Input: part model. Units: mm. Frame: model coordinates. A direction names the side the tool comes from. Round coordinates to 2 decimals unless told otherwise and drop trailing zeros. Write each loop counter-clockwise with the first axis right and the second up, starting at its lowest first coordinate (ties: lowest second). Pieces come first, ordered by that corner, then holes. Notation, with made-up numbers: (76.25, -13) -> (120.25, -13) arc R9 cw to (120.25, -4) -> close; hole circle Ø10 at (-35.5, 53.5). An arc over 180 degrees is marked (long way). Write item = value, one per line.
```python
from build123d import *

# Parameters (mm, degrees)
SKETCH1_R           = 5
BOSS_EXTRUDE1_DEPTH = 20
SKETCH2_R           = 2.5
CUT_EXTRUDE1_DEPTH  = 21
BOSS_EXTRUDE2_DEPTH = 18
SKETCH5_R           = 7.5
SKETCH5_R_2         = 2.5
BOSS_EXTRUDE3_DEPTH = 1
SKETCH4_R           = 7.5
BOSS_EXTRUDE4_DEPTH = 1
SKETCH7_R           = 0.5
CUT_EXTRUDE2_DEPTH  = 2


with BuildPart() as part:
    # Sketch1 → Boss-Extrude1 (new body)
    with BuildSketch(Plane(origin=(0, 0, 0), x_dir=(1, 0, 0), z_dir=(0, 1, 0))):
        with Locations(Location((0, 0, 0), (0, 0, 270))):  # turned: the seam where the file's is
            Circle(SKETCH1_R)
    extrude(amount=BOSS_EXTRUDE1_DEPTH)

    # Sketch2 → Cut-Extrude1 (cut, through all)
    with BuildSketch(Plane(origin=(0, 20, 0), x_dir=(1, 0, 0), z_dir=(0, 1, 0))):
        with Locations(Location((0, 0, 0), (0, 0, 270))):  # turned: the seam where the file's is
            Circle(SKETCH2_R)
    extrude(amount=-CUT_EXTRUDE1_DEPTH, mode=Mode.SUBTRACT)

    # Sketch3 → Boss-Extrude2 (add)
    with BuildSketch(Plane(origin=(0, 20, 0), x_dir=(1, 0, 0), z_dir=(0, 1, 0))):
        with BuildLine():
            Line((1.5, -2), (-1.5, -2))
            ThreePointArc((-1.5, -2), (0, -2.5), (1.5, -2))
        make_face()
    extrude(amount=-BOSS_EXTRUDE2_DEPTH)

    # Sketch5 → Boss-Extrude3 (add)
    with BuildSketch(Plane.XZ):
        with Locations(Location((0, 0, 0), (0, 0, 270))):  # turned: the seam where the file's is
            Circle(SKETCH5_R)
        with Locations(Location((0, 0, 0), (0, 0, 90))):  # turned: the seam where the file's is
            Circle(SKETCH5_R_2, mode=Mode.SUBTRACT)
    extrude(amount=-BOSS_EXTRUDE3_DEPTH)

    # Sketch4 → Boss-Extrude4 (add)
    with BuildSketch(Plane(origin=(0, 20, 0), x_dir=(1, 0, 0), z_dir=(0, 1, 0))):
        with Locations(Location((0, 0, 0), (0, 0, 90))):  # turned: the seam where the file's is
            Circle(SKETCH4_R)
        with BuildLine():
            Line((1.5, -2), (-1.5, -2))
            ThreePointArc((-1.5, -2), (0, 2.5), (1.5, -2))
        make_face(mode=Mode.SUBTRACT)
    extrude(amount=-BOSS_EXTRUDE4_DEPTH)

    # Sketch7 → Cut-Extrude2 (cut, through all)
    with BuildSketch(Plane.XZ.offset(-19)):
        with Locations(Location((-2.100852557, 5.628196829, 0), (0, 0, 270))):  # turned: the seam where the file's is
            Circle(SKETCH7_R)
    extrude(amount=-CUT_EXTRUDE2_DEPTH, mode=Mode.SUBTRACT)


solid = part.part
```
1) Cut plane B-B (z = 0). Return the cut outline in (x, y).
Solutions:
outline = (-7.5, 0) -> (-2.5, 0) -> (-2.5, 20) -> (-7.5, 20) -> (-7.5, 19) -> (-5, 19) -> (-5, 1) -> (-7.5, 1) -> close; (2.5, 0) -> (7.5, 0) -> (7.5, 1) -> (5, 1) -> (5, 19) -> (7.5, 19) -> (7.5, 20) -> (2.5, 20) -> close
2) Cut plane A-A (x = 0). Return the cut outline in (y, z).
Solutions:
outline = (0, -7.5) -> (1, -7.5) -> (1, -5) -> (19, -5) -> (19, -7.5) -> (20, -7.5) -> (20, -2.5) -> (0, -2.5) -> close; (0, 2.5) -> (2, 2.5) -> (2, 2) -> (20, 2) -> (20, 7.5) -> (19, 7.5) -> (19, 5) -> (1, 5) -> (1, 7.5) -> (0, 7.5) -> close
3) Cut plane C-C (y = 15). Return the cut outline in (x, z), and give its area (3 significant figures).
Solutions:
outline = circle Ø10 at (0, 0); hole (-1.5, 2) arc R2.5 ccw (long way) to (1.5, 2) -> close
area = 59.9 mm^2
4) Access query for faces 5 (the face through (-4.88, 9.87, -1.08)), 6 (the face through (0, 11, 2)), 7 (the face through (2, 0, 2)). Directions: +Z, -Z, +X, -X, +Y, -Y. A direction counts if a zero-diameter tool reaches every point of the face in a straight line with its end or side. Return the directions, or none.
Solutions:
face_5 = none
face_6 = +Y, -Y
face_7 = +Z, -Z, +X, -X, -Y
5) Cut plane D-D (x = 4.25). Return the cut outline in (y, z), and give its area (3 significant figures).
Solutions:
outline = (0, -6.18) -> (1, -6.18) -> (1, -2.63) -> (19, -2.63) -> (19, -6.18) -> (20, -6.18) -> (20, 6.18) -> (19, 6.18) -> (19, 2.63) -> (1, 2.63) -> (1, 6.18) -> (0, 6.18) -> close
area = 120 mm^2
6) First-contact query: P1, Ø6, axis at y = 13, z = 0, coming from the +X side; P2, Ø6, axis at y = 9.5, z = -4.5, coming from the -X side; P3, Ø4, axis at x = -5, y = 7.5, coming from the -Z side; P4, Ø3, axis at x = 0, z = 0, coming from the +Y side. Flat tips, straight axial feed; report the tip coordinate or a pass-through.
Solutions:
P1 = 5
P2 = -4.77
P3 = -4
P4 = through
7) Draft query along X for faces 1 (the face through (0.1, 10.1, -2.5)), 2 (the face through (-0.33, 19.507, 7.493)), 3 (the face through (-2, 20, 2)), 4 (the face through (-1.95, 19.49, 5.15)). Return one class per face: +X half, -X half, draft (parallel to the pull), parting line (faces both ways), or undercut.
Solutions:
face_1 = undercut
face_2 = parting line
face_3 = draft
face_4 = undercut
8) Line query: L1, parallel to Y at x = -5.75, z = -2; L2, parallel to X at y = 6.5, z = 0; L3, parallel to Z at x = 0, y = 3.5. Output: solid intervals per line, ascending. Write a range as from..to.
Solutions:
L1 = 0..1, 19..20
L2 = -5..-2.5, 2.5..5
L3 = -5..-2.5, 2..5
